from build123d import *

# Parameters (mm, degrees)
SKETCH1_W                = 76.2
SKETCH1_H                = 76.2
BOSS_EXTRUDE1_DEPTH      = 381
BOSS_EXTRUDE1_2_DEPTH    = 381
CUT_EXTRUDE1_DEPTH       = 945.678553795
CUT_EXTRUDE1_DEPTH_BACK  = 945.678553795
SKETCH3_W                = 28.047256614
SKETCH3_H                = 28.245033948
BOSS_EXTRUDE2_DEPTH      = 38.1
BOSS_EXTRUDE2_DEPTH_BACK = 38.1
SKETCH5_R                = 12.7
BOSS_EXTRUDE3_DEPTH      = 50.8


with BuildPart() as part:
    # Sketch1 → Boss-Extrude1 (new body)
    with BuildSketch(Plane(origin=(0, 0, 0), x_dir=(1, 0, 0), z_dir=(0, 1, 0))):
        Rectangle(SKETCH1_W, SKETCH1_H)
    extrude(amount=BOSS_EXTRUDE1_DEPTH)


with BuildPart() as body_2:
    # Sketch1 → Boss-Extrude1 2 (new body)
    with BuildSketch(Plane(origin=(0, 0, 0), x_dir=(1, 0, 0), z_dir=(0, 1, 0))):
        with Locations((-825.5, 0)):
            Rectangle(SKETCH1_W, SKETCH1_H)
    extrude(amount=BOSS_EXTRUDE1_2_DEPTH)


with BuildPart() as cut_extrude1_tool:
    # Sketch3 → Cut-Extrude1 (new, two sides: drawn at the far end of the back side and taken through both)
    with BuildSketch(Plane.XY.offset(-CUT_EXTRUDE1_DEPTH_BACK)):
        with Locations((-825.5, 39.522516974)):
            Rectangle(SKETCH3_W, SKETCH3_H)
        with Locations((0, 39.522516974)):
            Rectangle(SKETCH3_W, SKETCH3_H)
    extrude(amount=CUT_EXTRUDE1_DEPTH + CUT_EXTRUDE1_DEPTH_BACK)


with BuildPart() as part_1:
    add(part.part)

    # Cut-Extrude1: cut by cut_extrude1_tool
    add(cut_extrude1_tool.part, mode=Mode.SUBTRACT)



with BuildPart() as body_2_1:
    add(body_2.part)

    # Cut-Extrude1: cut by cut_extrude1_tool
    add(cut_extrude1_tool.part, mode=Mode.SUBTRACT)


with BuildPart() as part_2:
    add(part_1.part)

    add(body_2_1.part)  # Boss-Extrude2 merges body 2
    # Sketch4 → Boss-Extrude2 (add, two sides: drawn at the far end of the back side and taken through both)
    with BuildSketch(Plane.XY.offset(-BOSS_EXTRUDE2_DEPTH_BACK)):
        with BuildLine():
            Line((-863.6, 381), (-787.4, 381))
            ThreePointArc((-787.4, 381), (-412.75, 755.65), (-38.1, 381))
            Line((-38.1, 381), (38.1, 381))
            ThreePointArc((38.1, 381), (-412.75, 831.85), (-863.6, 381))
        make_face()
    extrude(amount=BOSS_EXTRUDE2_DEPTH + BOSS_EXTRUDE2_DEPTH_BACK)

    # Sketch5 → Boss-Extrude3 (add)
    with BuildSketch(Plane(origin=(0, 755.65, 0), x_dir=(1, 0, 0), z_dir=(0, 1, 0))):
        with Locations(Location((-412.75, 0, 0), (0, 0, 270))):
            Circle(SKETCH5_R)
    extrude(amount=-BOSS_EXTRUDE3_DEPTH)


solid = part_2.part
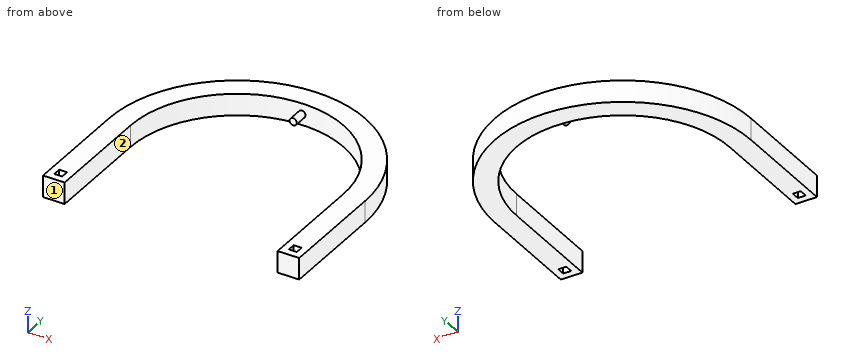
Input: part model. Units: mm. Frame: model coordinates. Face numbers are marked on the shaded views. A direction names the side the tool comes from. Give positions to 0.01 mm unless a question says otherwise; leave off trailing zeros. Write each loop counter-clockwise with the first axis right and the second up, starting at its lowest first coordinate (ties: lowest second). Pieces come first, ordered by that corner, then holes. Notation, with made-up numbers: M 60.25,64 L 80.25,64 A13 ccw 80.25,79 Z; hole C 70.25,65.25 d1. An arc over 180 degrees is marked long. Write item = value, one per line. Start each with the question number.
1) Material intervals for line 1 along X through (y, z) = (44.5, 8); line 2 along X through (y, z) = (125.5, -24.5); line 3 along Y through (x, z) = (-827, 23), sorted ascending. Write a range as [from, to].
2) Cut plane C-C on x = -412.75. Return the cut outline in (y, z).
3) First-contact query: pin 1 Ø10 at (y, z) = (554.5, -4) entering from +X; pin 2 Ø22.5 at (x, z) = (4.5, -9) entering from +Y (3 decimals); pin 3 Ø12 at (x, z) = (-178, -20.5) entering from +Y; pin 4 Ø22.5 at (x, z) = (1.5, -12.5) entering from -Y. Flat tips, straight axial feed; report the tip coordinate or a pass-through.
4) Cut plane A-A on y = 352. Return the cut outline in (x, z), then the cut area to 3 significant figures.
5) Cut plane D-D on x = -532. Return the cut outline in (y, z).
6) Reachability of the marked faces 1 and 2 from +Z, -Z, +X, -X, +Y, -Y: full face, straight path, thin tool, end or side. Return the list, or none.
7) Cut plane B-B on z = 24.5. Return the cut outline in (x, y).
Solved:
q1.line_1 = [-863.6, -839.52], [-811.48, -787.4], [-38.1, -14.02], [14.02, 38.1]
q1.line_2 = [-863.6, -787.4], [-38.1, 38.1]
q1.line_3 = [0, 25.4], [53.65, 558.94]
q2.outline = M 704.85,-12.7 L 755.65,-12.7 L 755.65,-38.1 L 831.85,-38.1 L 831.85,38.1 L 755.65,38.1 L 755.65,12.7 L 704.85,12.7 Z
q3.pin_1 = 5.43
q3.pin_2 = 577.035
q3.pin_3 = 769.51
q3.pin_4 = 0
q4.outline = M -863.6,-38.1 L -787.4,-38.1 L -787.4,38.1 L -863.6,38.1 Z; M -38.1,-38.1 L 38.1,-38.1 L 38.1,38.1 L -38.1,38.1 Z
q4.area = 11,600 mm2
q5.outline = M 736.16,-38.1 L 815.79,-38.1 L 815.79,38.1 L 736.16,38.1 Z
q6.face_1 = +Z, -Z, +X, -X, -Y
q6.face_2 = +Z, -Z, -Y
q7.outline = M -863.6,0 L -787.4,0 L -787.4,381 A374.65 cw -38.1,381 L -38.1,0 L 38.1,0 L 38.1,381 A450.85 ccw -863.6,381 Z; hole M -839.52,25.4 L -811.48,25.4 L -811.48,53.65 L -839.52,53.65 Z; hole M -14.02,25.4 L 14.02,25.4 L 14.02,53.65 L -14.02,53.65 Z
